```python
from build123d import *

# Parameters (mm, degrees)
BOSS_EXTRU_1_DEPTH = 10


with BuildPart() as part:
    # Esquisse1 → Boss.-Extru.1 (new body)
    with BuildSketch(Plane(origin=(0, 0, 0), x_dir=(1, 0, 0), z_dir=(0, 1, 0))):
        with BuildLine():
            Line((0, 5), (-38, 5))
            Line((-38, 5), (-38, -5))
            Line((-38, -5), (0, -5))
            ThreePointArc((0, -5), (5, 0), (0, 5))
        make_face()
    extrude(amount=BOSS_EXTRU_1_DEPTH)

    # Esquisse3 → Trou taraudé M61 (revolve, cut)
    with BuildSketch(Plane(origin=(0, 10, 0), x_dir=(0, 0, 1), z_dir=(1, 0, 0))):
        Polygon((0, 0), (0, 10), (3.5, 10), (2.5, 9), (2.5, 1), (3.5, 0), align=None)
    revolve(axis=Axis((0, 16.35, 0), (0, -1, 0)), mode=Mode.SUBTRACT)


solid = part.part
```
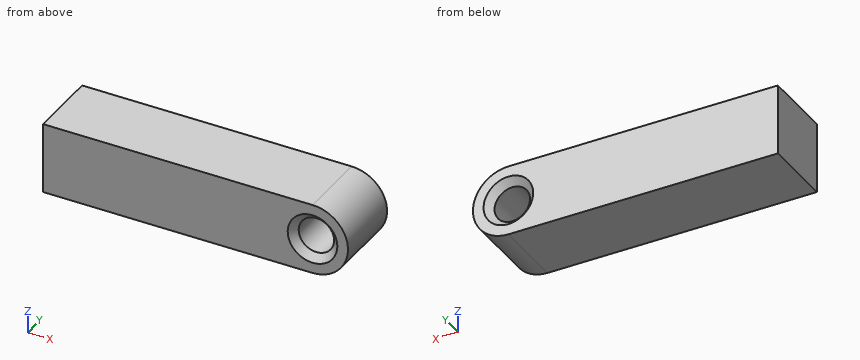
CAD build for the part. Positions are in the model's coordinates, mm. Coordinates: 2 decimals unless noted, no trailing zeros. Loops run counter-clockwise (first coordinate to the right, second up) from the corner with the lowest first, then second, coordinate; pieces in that order, holes last. Notation, with made-up numbers: (26.25, -11) - (46.25, -11) arc R21 cw to (46.25, 6) - close; hole circle Ø8 at (-11, 70.5). An arc over 180 degrees is marked (long way). Use CSV: the item, a comma, the result in double quotes. Start each with the question number.
Q1. Probe probe 1 along X at (y, z) = (4, 0); probe 2 along Z at (x, y) = (2, 9.5); probe 3 along X at (y, z) = (4.75, 1.75). List the from-to ranges inside material, lowest first. Write a range as from..to.
Q2. Cut at B-B, the plane y = 4. List the corners of the cut face in (x, z).
Q3. Cut at D-D, the plane z = 4.5. List the corners of the cut face in (x, y), then the cut area to 3 significant figures.
Q4. Cut at C-C, the plane y = 9.5. List the corners of the cut face in (x, z), then the cut area to 3 significant figures.
Q5. Cut at A-A, the plane z = 0. List the corners of the cut face in (x, y), then the cut area to 3 significant figures.
Here are the results:
1,probe 1,"-38..-2.5, 2.5..5"
1,probe 2,"-4.58..-2.24, 2.24..4.58"
1,probe 3,"-38..-1.79, 1.79..4.68"
2,outline,"(-38, -5) - (0, -5) arc R5 ccw to (0, 5) - (-38, 5) - close; hole circle Ø5 at (0, 0)"
3,outline,"(-38, 0) - (2.18, 0) - (2.18, 10) - (-38, 10) - close"
3,area,"402 mm2"
4,outline,"(-38, -5) - (0, -5) arc R5 ccw to (0, 5) - (-38, 5) - close; hole circle Ø6 at (0, 0)"
4,area,"391 mm2"
5,outline,"(-38, 0) - (-3.5, 0) - (-2.5, 1) - (-2.5, 9) - (-3.5, 10) - (-38, 10) - close; (2.5, 1) - (3.5, 0) - (5, 0) - (5, 10) - (3.5, 10) - (2.5, 9) - close"
5,area,"378 mm2"
